from build123d import *

# Parameters (mm, degrees)
F0_R     = 1.5
F0_R_2   = 2
F0_R_3   = 25.5
F1_DEPTH = 10
F2_R     = 0.5
F3_DEPTH = 15
F4_R     = 0.5
F5_DEPTH = 15
F6_R     = 0.5
F7_DEPTH = 15


with BuildPart() as f1:
    # F0 (on Top) → F1 (new body)
    with BuildSketch(Plane.XY):
        with BuildLine():
            Line((-32.371039, -11.931716), (-26.518689, -22.068284))
            ThreePointArc((-26.518689, -22.068284), (0, -34.5), (26.518689, -22.068284))
            Line((26.518689, -22.068284), (32.371039, -11.931716))
            ThreePointArc((32.371039, -11.931716), (29.877876, 17.25), (5.85235, 34))
            Line((5.85235, 34), (-5.85235, 34))
            ThreePointArc((-5.85235, 34), (-29.877876, 17.25), (-32.371039, -11.931716))
        make_face()
        with Locations((-19.283628, -22.981333)):
            Circle(F0_R, mode=Mode.SUBTRACT)
        with Locations((-10.260604, -28.190779)):
            Circle(F0_R, mode=Mode.SUBTRACT)
        with Locations((-25.980762, -15)):
            Circle(F0_R_2, mode=Mode.SUBTRACT)
        with Locations((-29.544233, -5.209445)):
            Circle(F0_R, mode=Mode.SUBTRACT)
        with Locations((0, -30)):
            Circle(F0_R, mode=Mode.SUBTRACT)
        with Locations((10.260604, -28.190779)):
            Circle(F0_R, mode=Mode.SUBTRACT)
        with Locations((19.283628, -22.981333)):
            Circle(F0_R, mode=Mode.SUBTRACT)
        with Locations((25.980762, -15)):
            Circle(F0_R_2, mode=Mode.SUBTRACT)
        with Locations((29.544233, -5.209445)):
            Circle(F0_R, mode=Mode.SUBTRACT)
        with Locations((-29.544233, 5.209445)):
            Circle(F0_R, mode=Mode.SUBTRACT)
        with Locations((-25.980762, 15)):
            Circle(F0_R, mode=Mode.SUBTRACT)
        with Locations((-19.283628, 22.981333)):
            Circle(F0_R, mode=Mode.SUBTRACT)
        with Locations((-10.260604, 28.190779)):
            Circle(F0_R, mode=Mode.SUBTRACT)
        Circle(F0_R_3, mode=Mode.SUBTRACT)
        with Locations((29.544233, 5.209445)):
            Circle(F0_R, mode=Mode.SUBTRACT)
        with Locations((25.980762, 15)):
            Circle(F0_R, mode=Mode.SUBTRACT)
        with Locations((0, 30)):
            Circle(F0_R_2, mode=Mode.SUBTRACT)
        with Locations((10.260604, 28.190779)):
            Circle(F0_R, mode=Mode.SUBTRACT)
        with Locations((19.283628, 22.981333)):
            Circle(F0_R, mode=Mode.SUBTRACT)
    extrude(amount=F1_DEPTH)

    # F2 (on face) → F3 (cut)
    with BuildSketch(Plane(origin=(29.444864, -17, 0), x_dir=(0.5, 0.866025, 0), z_dir=(0.866025, -0.5, 0))):
        with Locations((0, 5)):
            Circle(F2_R)
    extrude(amount=-F3_DEPTH, mode=Mode.SUBTRACT)

    # F4 (on face) → F5 (cut)
    with BuildSketch(Plane(origin=(0, 34, 0), x_dir=(-1, 0, 0), z_dir=(0, 1, 0))):
        with Locations((0, 5)):
            Circle(F4_R)
    extrude(amount=-F5_DEPTH, mode=Mode.SUBTRACT)

    # F6 (on face) → F7 (cut)
    with BuildSketch(Plane(origin=(-29.444864, -17, 0), x_dir=(0.5, -0.866025, 0), z_dir=(-0.866025, -0.5, 0))):
        with Locations((0, 5)):
            Circle(F6_R)
    extrude(amount=-F7_DEPTH, mode=Mode.SUBTRACT)


solid = f1.part
Input: part model. Units: mm. Frame: model coordinates. Coordinates: 2 decimals unless noted, no trailing zeros. Loops run counter-clockwise (first coordinate to the right, second up) from the corner with the lowest first, then second, coordinate; pieces in that order, holes last.
Q1. Cut plane B-B (y = 15). Output: boundary loops of the cut face in (x, z).
Q2. Cut plane D-D (x = -15). Output: boundary loops of the cut face in (y, z), then the cut area to 3 significant figures.
Q3. Contact query for flat-ended pins moving along their axis: pin 1 (2.5 mm diameter, centred on x = -19.28, y = 22.98, fed in from -Z); pin 2 (3 mm diameter, centred on y = 5, z = 2, fed in from -X); pin 3 (1 mm diameter, centred on x = -22, z = 5, fed in from +Y). Output: stop coordinate, or through.
Q4. Material intervals for line 1 (X direction, y = 15.5, z = 2.25); line 2 (Y direction, x = 30, z = 1); line 3 (Y direction, x = 10, z = 1), sorted ascending.
Q5. Draft query along X for faces 1 (the face through (0, 34, 6)), 2 (the face through (-29.66, 17.62, 4.93)), 3 (the face through (-17.853, -22.531, 4.93)). Return one class per face: +X half, -X half, draft (parallel to the pull), parting line (faces both ways), or undercut.
Q6. Cut plane C-C (z = 8.25). Give the number of separate pieces and of enclosed holes in the cut face, then the cut area to 3 significant figures.
Q7. Cut plane A-A (y = 0). Output: boundary loops of the cut face in (x, z).
Working result:
1. outline: (-31.07, 0) - (-27.48, 0) - (-27.48, 10) - (-31.07, 10) - close; (-24.48, 0) - (-20.62, 0) - (-20.62, 10) - (-24.48, 10) - close; (20.62, 0) - (24.48, 0) - (24.48, 10) - (20.62, 10) - close; (27.48, 0) - (31.07, 0) - (31.07, 10) - (27.48, 10) - close
2. outline: (-31.07, 0) - (-20.62, 0) - (-20.62, 10) - (-31.07, 10) - close; (20.62, 0) - (31.07, 0) - (31.07, 10) - (20.62, 10) - close
2. area: 209 mm2
3. pin 1: passes through
3. pin 2: stops at x = -34.32
3. pin 3: stops at y = 26.98
4. line 1: x = -30.82 to -27.39, -24.57 to -20.25, 20.25 to 24.57, 27.39 to 30.82
4. line 2: y = -16.04 to -6.64, -3.78 to 3.78, 6.64 to 17.04
4. line 3: y = -33.02 to -29.67, -26.71 to -23.46, 23.46 to 26.71, 29.67 to 33.02
5. face 1: draft
5. face 2: -X half
5. face 3: undercut
6. separate pieces: 1
6. enclosed holes: 19
6. area: 1,540 mm2
7. outline: (-34.5, 0) - (-25.5, 0) - (-25.5, 10) - (-34.5, 10) - close; (25.5, 0) - (34.5, 0) - (34.5, 10) - (25.5, 10) - close
